```python
from build123d import *

# Parameters (mm, degrees)
SKETCH1_R           = 3.937
SKETCH1_R_2         = 0.4445
SKETCH1_W           = 3.2258
SKETCH1_H           = 6.35
BOSS_EXTRUDE1_DEPTH = 3.175
BOSS_EXTRUDE2_DEPTH = 3.175
CUT_EXTRUDE1_DEPTH  = 4.175


with BuildPart() as part:
    # Sketch1 → Boss-Extrude1 (new body)
    with BuildSketch(Plane(origin=(0, 0, 0), x_dir=(0, 0, -1), z_dir=(1, 0, 0))):
        Polygon((-6.985, 7.62), (6.985, 7.62), (6.985, -22.606), (-33.782, -22.606), (-33.782, -16.256), (-37.0078, -16.256), (-37.0078, -9.906), (-33.782, -9.906), (-33.782, -7.366), (-27.94, -7.366), (-27.94, -16.764), (-18.796, -16.764), (-18.796, -7.366), (-6.985, -7.366), align=None)
        Circle(SKETCH1_R, mode=Mode.SUBTRACT)
        with Locations((2.40063044, -6.111302341)):
            Circle(SKETCH1_R_2, mode=Mode.SUBTRACT)
        with Locations((4.490066454, -11.430652127)):
            Circle(SKETCH1_R_2, mode=Mode.SUBTRACT)
        with Locations((-10.5791, -14.351)):
            Rectangle(SKETCH1_W, SKETCH1_H, mode=Mode.SUBTRACT)
    extrude(amount=BOSS_EXTRUDE1_DEPTH)

    # Sketch2 → Boss-Extrude2 (add)
    with BuildSketch(Plane.ZY):
        Polygon((13.462, -23.876), (31.582295474, -23.876), (33.782, -22.606), (12.192, -22.606), align=None)
    extrude(amount=-BOSS_EXTRUDE2_DEPTH)

    # Sketch3 → Cut-Extrude1 (cut, through all)
    with BuildSketch(Plane(origin=(3.175, 0, 0), x_dir=(0, 0, -1), z_dir=(1, 0, 0))):
        Polygon((-30.861, -7.366), (-27.94, -7.366), (-27.94, -12.065), align=None)
        with BuildLine():
            Line((6.985, -13.716), (6.985, -22.606))
            Line((6.985, -22.606), (0.635, -22.606))
            ThreePointArc((0.635, -22.606), (4.50973023, -18.660807307), (6.985, -13.716))
        make_face()
    extrude(amount=-CUT_EXTRUDE1_DEPTH, mode=Mode.SUBTRACT)


solid = part.part
```
Input: part model. Units: mm. Frame: model coordinates. A direction names the side the tool comes from. Round coordinates to 2 decimals unless told otherwise and drop trailing zeros. Loops run counter-clockwise (first coordinate to the right, second up) from the corner with the lowest first, then second, coordinate; pieces in that order, holes last. Notation, with made-up numbers: (47.25, 30.25) -> (102.25, 30.25) arc R32 ccw to (102.25, 61.25) -> close; hole circle Ø8 at (10, -22.5). An arc over 180 degrees is marked (long way). Write each question's results on one line, items separated by ' | '.
1. Section A-A (y = 0). Return loops of the section in (x, z) (3 decimals), and give its area (3 significant figures).
Geometry results:
outline: (0, -6.985) -> (3.175, -6.985) -> (3.175, -3.937) -> (0, -3.937) -> close; (0, 3.937) -> (3.175, 3.937) -> (3.175, 6.985) -> (0, 6.985) -> close | area: 19.4 mm2
2. Set-up query: faces 1 (the face through (2, -14, 12.192)), 2 (the face through (2, -22.606, 6)), 3 (the face through (2, 0, 6.985)), 4 (the face through (2, -16.764, 23)). Return all of +Z, -Z, +X, -X, +Y, -Y with unobstructed straight access to the full face (end or side cutting, diameter ignored); none if empty.
Geometry results:
face 1: +X, -X | face 2: -Z, +X, -X, -Y | face 3: +Z, +X, -X, +Y | face 4: +X, -X, +Y
3. Mould query, pull axis Z, two halves, no side actions, for faces 5 (the face through (2, -16.256, 35)), 6 (the face through (2, -9, 33.782)), 7 (the face through (2, -14, 27.94)). Classes: +Z half, -Z half, draft (parallel to the pull), parting line (faces both ways), or undercut.
Geometry results:
face 5: draft | face 6: +Z half | face 7: undercut
4. Section D-D (z = 5). Return loops of the section in (x, y) (3 decimals).
Geometry results:
outline: (0, -22.606) -> (3.175, -22.606) -> (3.175, 7.62) -> (0, 7.62) -> close
5. First-contact query: P1, Ø1.6, axis at x = 1.5, y = 3.5, coming from the +Z side (3 decimals); P2, Ø1.5, axis at x = 2, z = 31.5, coming from the +Y side; P3, Ø1.5, axis at x = 1, z = 25.5, coming from the +Y side; P4, Ø4, axis at y = -11.5, z = 5.5, coming from the -X side. Flat tips, straight axial feed; report the tip coordinate or a pass-through.
Geometry results:
P1: z = 6.985 | P2: y = -7.37 | P3: y = -16.76 | P4: x = 0
6. Section C-C (x = 0.75). Return loops of the section in (y, z) (1 decimal), and give its area (3 significant figures).
Geometry results:
outline: (-23.9, 13.5) -> (-22.6, 12.2) -> (-22.6, -0.6) arc R17.8 ccw to (-13.7, -7) -> (7.6, -7) -> (7.6, 7) -> (-7.4, 7) -> (-7.4, 18.8) -> (-16.8, 18.8) -> (-16.8, 27.9) -> (-12.1, 27.9) -> (-7.4, 30.9) -> (-7.4, 33.8) -> (-9.9, 33.8) -> (-9.9, 37) -> (-16.3, 37) -> (-16.3, 33.8) -> (-22.6, 33.8) -> (-23.9, 31.6) -> close; hole (-17.5, 9) -> (-11.2, 9) -> (-11.2, 12.2) -> (-17.5, 12.2) -> close; hole circle Ø0.9 at (-11.4, -4.5); hole circle Ø0.9 at (-6.1, -2.4); hole circle Ø7.9 at (0, 0) | area: 691 mm2
7. Ray query, line 1 (Y direction, x = 0.95, z = 0); line 2 (Y direction, x = 2.25, z = 26); line 3 (Y direction, x = 1.1, z = 8). Return the intervals inside material, ascending. Write a range as from..to.
Geometry results:
line 1: -22.61..-3.94, 3.94..7.62 | line 2: -23.88..-16.76 | line 3: -22.61..-7.37
8. Section B-B (z = 0). Return loops of the section in (x, y) (3 decimals), and give its area (3 significant figures).
Geometry results:
outline: (0, -22.606) -> (3.175, -22.606) -> (3.175, -3.937) -> (0, -3.937) -> close; (0, 3.937) -> (3.175, 3.937) -> (3.175, 7.62) -> (0, 7.62) -> close | area: 71.0 mm2
